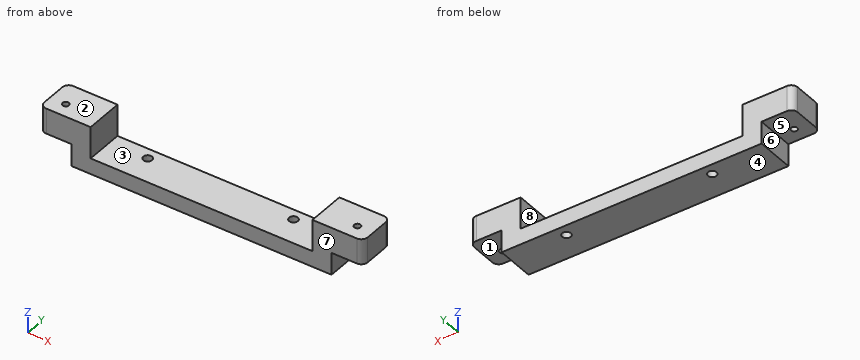
from build123d import *

# Parameters (mm, degrees)
F1_DEPTH      = 15
F2_W          = 70
F2_H          = 12
F3_DEPTH      = 10
F4_R          = 1.375
F4_R_2        = 1
F5_DEPTH      = 25
F5_DEPTH_BACK = 25
F6_R          = 1
F7_DEPTH      = 7


with BuildPart() as f1:
    # F0 (on Top) → F1 (new body)
    with BuildSketch(Plane.XY):
        with BuildLine():
            ThreePointArc((-15.4861029406, 2), (-14.9003165029, 0.5857864376), (-13.4861029406, 0))
            Line((-13.4861029406, 0), (84.5138970594, 0))
            ThreePointArc((84.5138970594, 0), (85.9281106218, 0.5857864376), (86.5138970594, 2))
            Line((86.5138970594, 2), (86.5138970594, 10))
            ThreePointArc((86.5138970594, 10), (85.9281106218, 11.4142135624), (84.5138970594, 12))
            Line((84.5138970594, 12), (-13.4861029406, 12))
            ThreePointArc((-13.4861029406, 12), (-14.9003165029, 11.4142135624), (-15.4861029406, 10))
            Line((-15.4861029406, 10), (-15.4861029406, 2))
        make_face()
    extrude(amount=F1_DEPTH)

    # F2 (on face) → F3 (cut)
    with BuildSketch(Plane.XY.offset(15)):
        with Locations((35.5138970594, 6)):
            Rectangle(F2_W, F2_H)
    extrude(amount=-F3_DEPTH, mode=Mode.SUBTRACT)

    # F4 (on face) → F5 (cut, two sides)
    with BuildSketch(Plane.XY.offset(5)) as f5_sk:
        with Locations((12.5138970594, 8.5)):
            Circle(F4_R)
        with Locations((58.5138970594, 8.5)):
            Circle(F4_R)
        with Locations((-10.4861029406, 4.5)):
            Circle(F4_R_2)
        with Locations((81.5138970594, 4.5)):
            Circle(F4_R_2)
    extrude(amount=-F5_DEPTH, mode=Mode.SUBTRACT)
    extrude(f5_sk.sketch, amount=F5_DEPTH_BACK, mode=Mode.SUBTRACT)

    # F6 (on face) → F7 (cut)
    with BuildSketch(Plane(origin=(0, 0, 0), x_dir=(1, 0, 0), z_dir=(0, 0, -1))):
        with BuildLine():
            Line((76.5138970594, 0), (76.5138970594, -12))
            Line((76.5138970594, -12), (84.5138970594, -12))
            ThreePointArc((84.5138970594, -12), (85.9281106218, -11.4142135624), (86.5138970594, -10))
            Line((86.5138970594, -10), (86.5138970594, -2))
            ThreePointArc((86.5138970594, -2), (85.9281106218, -0.5857864376), (84.5138970594, 0))
            Line((84.5138970594, 0), (76.5138970594, 0))
        make_face()
        with Locations((81.5138970594, -4.5)):
            Circle(F6_R, mode=Mode.SUBTRACT)
        with BuildLine():
            Line((-13.4861029406, -12), (-5.4861029406, -12))
            Line((-5.4861029406, -12), (-5.4861029406, 0))
            Line((-5.4861029406, 0), (-13.4861029406, 0))
            ThreePointArc((-13.4861029406, 0), (-14.9003165029, -0.5857864376), (-15.4861029406, -2))
            Line((-15.4861029406, -2), (-15.4861029406, -10))
            ThreePointArc((-15.4861029406, -10), (-14.9003165029, -11.4142135624), (-13.4861029406, -12))
        make_face()
        with Locations((-10.4861029406, -4.5)):
            Circle(F6_R, mode=Mode.SUBTRACT)
    extrude(amount=-F7_DEPTH, mode=Mode.SUBTRACT)


solid = f1.part
Build history of the part. All positions in model axes, mm. Face numbers are marked on the shaded views. A direction names the side the tool comes from. Round coordinates to 2 decimals unless told otherwise and drop trailing zeros. Write each loop counter-clockwise with the first axis right and the second up, starting at its lowest first coordinate (ties: lowest second). Pieces come first, ordered by that corner, then holes. Notation, with made-up numbers: (36, 35) - (91, 35) arc R33 ccw to (91, 71) - close; hole circle Ø2 at (-26, 33). An arc over 180 degrees is marked (long way). Use CSV: the item, a comma, the result in double quotes.
(1) Band-saw the part on C-C (z = 3.25). Write the cut outline in (x, y) (3 decimals), plus the area to 3 significant figures.
Response:
outline,"(-5.486, 0) - (76.514, 0) - (76.514, 12) - (-5.486, 12) - close; hole circle Ø2.75 at (12.514, 8.5); hole circle Ø2.75 at (58.514, 8.5)"
area,"972 mm²"
(2) Band-saw the part on D-D (y = 4.5). Write the cut outline in (x, z), plus the area to 3 significant figures.
Response:
outline,"(-15.49, 7) - (-11.49, 7) - (-11.49, 15) - (-15.49, 15) - close; (-9.49, 7) - (-5.49, 7) - (-5.49, 0) - (76.51, 0) - (76.51, 7) - (80.51, 7) - (80.51, 15) - (70.51, 15) - (70.51, 5) - (0.51, 5) - (0.51, 15) - (-9.49, 15) - close; (82.51, 7) - (86.51, 7) - (86.51, 15) - (82.51, 15) - close"
area,"658 mm²"
(3) Mould opens along X. For the marked faces 6, 7 and 8 say: pulls with the +X half, pulls with the -X half, needs draft (parallel to the pull), parting line crosses it, or undercut.
Response:
face 6,"pulls with the -X half"
face 7,"needs draft"
face 8,"undercut"
(4) Band-saw the part on A-A (z = 10.5). Write the cut outline in (x, y), plus the area to 3 significant figures.
Response:
outline,"(-15.49, 2) arc R2 ccw to (-13.49, 0) - (0.51, 0) - (0.51, 12) - (-13.49, 12) arc R2 ccw to (-15.49, 10) - close; (70.51, 0) - (84.51, 0) arc R2 ccw to (86.51, 2) - (86.51, 10) arc R2 ccw to (84.51, 12) - (70.51, 12) - close; hole circle Ø2 at (-10.49, 4.5); hole circle Ø2 at (81.51, 4.5)"
area,"374 mm²"
(5) 3-axis set-ups, long thin cutter, end or side, ignore diameter. For the marked faces 1, 2, 3, 4 and 5: which of +Z, -Z, +X, -X, +Y, -Y reach the whole face in a straight line?
Response:
face 1,"-Z, +X, +Y, -Y"
face 2,"+Z, +X, -X, +Y, -Y"
face 3,"+Z, +Y, -Y"
face 4,"-Z, +X, -X, +Y, -Y"
face 5,"-Z, -X, +Y, -Y"
(6) Wall check: line 1 (X direction, y = 4.5, z = 9.25); line 2 (X direction, y = 10.25, z = 7.5); line 3 (Z direction, x = -6.5, y = 9.5). Give the ranges that are in metal, low to high.
Response:
line 1,"-15.49 to -11.49, -9.49 to 0.51, 70.51 to 80.51, 82.51 to 86.51"
line 2,"-15.47 to 0.51, 70.51 to 86.5"
line 3,"7 to 15"
(7) Band-saw the part on B-B (y = 8.5). Write the cut outline in (x, z), plus the area to 4 significant figures.
Response:
outline,"(-15.49, 7) - (-5.49, 7) - (-5.49, 0) - (11.14, 0) - (11.14, 5) - (0.51, 5) - (0.51, 15) - (-15.49, 15) - close; (13.89, 0) - (57.14, 0) - (57.14, 5) - (13.89, 5) - close; (59.89, 0) - (76.51, 0) - (76.51, 7) - (86.51, 7) - (86.51, 15) - (70.51, 15) - (70.51, 5) - (59.89, 5) - close"
area,"662.5 mm²"
(8) Pin check, flat tips, straight feed: P1, Ø6, axis at y = 4.5, z = 2.5, coming from the -X side; P2, Ø3.5, axis at x = 28, y = 6.5, coming from the +Z side; P3, Ø1, axis at y = 3.5, z = 2.5, coming from the +X side; P4, Ø2.5, axis at x = 12.51, y = 8.5, coming from the -Z side. Stop position of each tip, or through.
Response:
P1,"x = -5.49"
P2,"z = 5"
P3,"x = 76.51"
P4,"through"
